Build history of the part. All positions in model axes, mm. A direction names the side the tool comes from. Coordinates: 2 decimals unless noted, no trailing zeros. Write each loop counter-clockwise with the first axis right and the second up, starting at its lowest first coordinate (ties: lowest second). Pieces come first, ordered by that corner, then holes.
```python
from build123d import *

# Parameters (mm, degrees)
SKETCH1_W                = 16.2
SKETCH1_H                = 8.4
BOSS_EXTRUDE1_DEPTH      = 14.5
SKETCH3_R                = 1.9
BOSS_EXTRUDE2_DEPTH      = 3
SKETCH3_3_R              = 1.9
BOSS_EXTRUDE3_DEPTH      = 6
SKETCH6_W                = 3.5
SKETCH6_H                = 8.4
SKETCH6_R                = 1
BOSS_EXTRUDE4_DEPTH      = 0.6
FILLET2_START            = -1
FILLET2_DEPTH            = 19
FILLET3_START            = -1
FILLET3_DEPTH            = 16
BOSS_EXTRUDE5_DEPTH      = 0.6
SKETCH8_W                = 3.8
SKETCH8_H                = 4
BOSS_EXTRUDE6_DEPTH      = 0.6
CHAMFER1_SIZE            = 1
M2_CLEARANCE_HOLE1_D     = 2.4
M2_CLEARANCE_HOLE1_DEPTH = 6
M2_CLEARANCE_HOLE1_TIP   = 0.721032743


with BuildPart() as part:
    # Sketch1 → Boss-Extrude1 (new body)
    with BuildSketch(Plane(origin=(0, 0, 0), x_dir=(1, 0, 0), z_dir=(0, 1, 0))):
        Rectangle(SKETCH1_W, SKETCH1_H)
    extrude(amount=BOSS_EXTRUDE1_DEPTH)

    # Sketch3 → Boss-Extrude2 (add)
    with BuildSketch(Plane(origin=(0, 14.5, 0), x_dir=(1, 0, 0), z_dir=(0, 1, 0))):
        with BuildLine():
            Line((3.9, 4.2), (8.1, 4.2))
            Line((8.1, 4.2), (8.1, -4.2))
            Line((8.1, -4.2), (3.9, -4.2))
            ThreePointArc((3.9, -4.2), (1.840026431, -3.660124164), (0.309638554, -2.179289951))
            ThreePointArc((0.309638554, -2.179289951), (-2.5, 0), (0.309638554, 2.179289951))
            ThreePointArc((0.309638554, 2.179289951), (1.840026431, 3.660124164), (3.9, 4.2))
        make_face()
        with Locations(Location((3.9, 0, 0), (0, 0, 270))):
            Circle(SKETCH3_R, mode=Mode.SUBTRACT)
    extrude(amount=BOSS_EXTRUDE2_DEPTH)

    # Sketch3<3> → Boss-Extrude3 (add)
    with BuildSketch(Plane(origin=(0, 14.5, 0), x_dir=(1, 0, 0), z_dir=(0, 1, 0))):
        with Locations(Location((3.9, 0, 0), (0, 0, 270))):
            Circle(SKETCH3_3_R)
    extrude(amount=BOSS_EXTRUDE3_DEPTH)

    # Sketch6 → Boss-Extrude4 (add)
    # profile 1 of 2: a face of its own
    with BuildSketch(Plane(origin=(0, 8, 0), x_dir=(1, 0, 0), z_dir=(0, 1, 0))):
        with Locations((9.85, 0)):
            Rectangle(SKETCH6_W, SKETCH6_H)
        with Locations(Location((9.75, 0, 0), (0, 0, 270))):
            Circle(SKETCH6_R, mode=Mode.SUBTRACT)
    # profile 2 of 2: a face of its own
    with BuildSketch(Plane(origin=(0, 8, 0), x_dir=(1, 0, 0), z_dir=(0, 1, 0))):
        with Locations((-9.85, 0)):
            Rectangle(SKETCH6_W, SKETCH6_H)
        with Locations(Location((-9.75, 0, 0), (0, 0, 90))):
            Circle(SKETCH6_R, mode=Mode.SUBTRACT)
    extrude(amount=BOSS_EXTRUDE4_DEPTH)

    # Fillet2: read off the stored shape, not the designer's step
    # Fillet2 outline → Fillet2 (cut)
    with BuildSketch(Plane(origin=(0, 0, 0), x_dir=(1, 0, 0), z_dir=(0, 1, 0)).offset(FILLET2_START)):
        with BuildLine():
            ThreePointArc((7.4, 4.2), (10.369848481, 2.969848481), (11.6, 0))
            Line((11.6, 0), (11.6, 4.2))
            Line((11.6, 4.2), (7.4, 4.2))
        make_face()
        with BuildLine():
            Line((11.6, -4.2), (11.6, 0))
            ThreePointArc((11.6, 0), (10.369848481, -2.969848481), (7.4, -4.2))
            Line((7.4, -4.2), (11.6, -4.2))
        make_face()
    extrude(amount=FILLET2_DEPTH, mode=Mode.SUBTRACT)

    # Fillet3: read off the stored shape, not the designer's step
    # Fillet3 outline → Fillet3 (cut)
    with BuildSketch(Plane(origin=(0, 0, 0), x_dir=(1, 0, 0), z_dir=(0, 1, 0)).offset(FILLET3_START)):
        with BuildLine():
            ThreePointArc((-7.4, -4.2), (-10.369848481, -2.969848481), (-11.6, 0))
            Line((-11.6, 0), (-11.6, -4.2))
            Line((-11.6, -4.2), (-7.4, -4.2))
        make_face()
        with BuildLine():
            Line((-11.6, 4.2), (-11.6, 0))
            ThreePointArc((-11.6, 0), (-10.369848481, 2.969848481), (-7.4, 4.2))
            Line((-7.4, 4.2), (-11.6, 4.2))
        make_face()
    extrude(amount=FILLET3_DEPTH, mode=Mode.SUBTRACT)

    # Sketch7 → Boss-Extrude5 (add)
    with BuildSketch(Plane(origin=(0, 17.5, 0), x_dir=(1, 0, 0), z_dir=(0, 1, 0))):
        with BuildLine():
            Line((-1.05, 1), (0.4, 1))
            ThreePointArc((0.4, 1), (1.4, 0), (0.4, -1))
            Line((0.4, -1), (-1.05, -1))
            ThreePointArc((-1.05, -1), (-2.05, 0), (-1.05, 1))
        make_face()
    extrude(amount=BOSS_EXTRUDE5_DEPTH)

    # Sketch8 → Boss-Extrude6 (add)
    with BuildSketch(Plane(origin=(8.1, 0, 0), x_dir=(0, 0, -1), z_dir=(1, 0, 0))):
        with Locations((0, 2)):
            Rectangle(SKETCH8_W, SKETCH8_H)
    extrude(amount=BOSS_EXTRUDE6_DEPTH)

    # Chamfer1
    chamfer1_edges = [part.edges().sort_by_distance(p)[0] for p in [
        (-8.1, 14.5, 0),
    ]]
    chamfer(chamfer1_edges, length=CHAMFER1_SIZE)

    # M2 Clearance Hole1
    with Locations(Plane(origin=(0, 20.5, 0), x_dir=(1, 0, 0), z_dir=(0, 1, 0))):
        with Locations((3.9, 0)):
            Hole(M2_CLEARANCE_HOLE1_D / 2, depth=M2_CLEARANCE_HOLE1_DEPTH)
            with Locations((0, 0, -(M2_CLEARANCE_HOLE1_DEPTH + M2_CLEARANCE_HOLE1_TIP / 2))):  # 118° drill point
                Cone(0, M2_CLEARANCE_HOLE1_D / 2, M2_CLEARANCE_HOLE1_TIP, mode=Mode.SUBTRACT)


solid = part.part
```
1. 3-axis set-ups, long thin cutter, end or side, ignore diameter. For faces 4 (the face through (8.7, 2, 0)), 5 (the face through (-8.1, 4, 0)), 6 (the face through (2.755, 17.458, -0.36)): which of +Z, -Z, +X, -X, +Y, -Y reach the whole face in a straight line?
Computed values:
face 4: +Z, -Z, +X, -Y
face 5: +Z, -Z, -X, -Y
face 6: +Y
2. Saw through at A-A on y = 2.25. List the corners of the cut face in (x, z).
Computed values:
outline: (-8.1, -4.14) arc R4.2 ccw to (-7.4, -4.2) - (7.4, -4.2) arc R4.2 ccw to (8.1, -4.14) - (8.1, -1.9) - (8.7, -1.9) - (8.7, 1.9) - (8.1, 1.9) - (8.1, 4.14) arc R4.2 ccw to (7.4, 4.2) - (-7.4, 4.2) arc R4.2 ccw to (-8.1, 4.14) - close
3. Mould opens along X. For faces 1 (the face through (8.1, 13, 0)), 2 (the face through (-2.05, 17.8, 0.02)), 3 (the face through (10.74, 8.3, -0.13)) say: +X half, -X half, draft (parallel to the pull), parting line (faces both ways), or undercut.
Computed values:
face 1: +X half
face 2: -X half
face 3: undercut
4. Saw through at D-D on z = -1.5. List the corners of the cut face in (x, y), plus the area to 3 significant figures.
Computed values:
outline: (-11.32, 8) - (-8.1, 8) - (-8.1, 0) - (8.7, 0) - (8.7, 4) - (8.1, 4) - (8.1, 8) - (11.32, 8) - (11.32, 8.6) - (8.1, 8.6) - (8.1, 17.5) - (5.07, 17.5) - (5.07, 20.5) - (2.73, 20.5) - (2.73, 17.5) - (-1.93, 17.5) - (-1.93, 14.5) - (-7.1, 14.5) - (-8.1, 13.5) - (-8.1, 8.6) - (-11.32, 8.6) - close
area: 278 mm2
5. Flat gauge pins, fed straight in: pin 1 (2 mm diameter, centred on x = -5, z = -3, fed in from -Y); pin 2 (1 mm diameter, centred on y = 12.5, z = 0, fed in from -X); pin 3 (1 mm diameter, centred on x = -10, z = 1, fed in from -Y); pin 4 (2.5 mm diameter, centred on x = -9.75, z = 0, fed in from +Y). Where does each tip first touch, or does it go through?
Computed values:
pin 1: stops at y = 0
pin 2: stops at x = -8.1
pin 3: stops at y = 8
pin 4: stops at y = 8.6
6. Probe line 1 along X through (y, z) = (10, 2.75); line 2 along Y through (x, z) = (2.25, -2); line 3 along Y through (x, z) = (-6, -0.5). List the from-to ranges inside material, lowest first.
Computed values:
line 1: x = -8.1 to 8.1
line 2: y = 0 to 17.5
line 3: y = 0 to 14.5
7. Saw through at B-B on x = -0.25. List the corners of the cut face in (y, z).
Computed values:
outline: (0, -4.2) - (14.5, -4.2) - (14.5, -2.25) - (17.5, -2.25) - (17.5, -1) - (18.1, -1) - (18.1, 1) - (17.5, 1) - (17.5, 2.25) - (14.5, 2.25) - (14.5, 4.2) - (0, 4.2) - close
8. Saw through at C-C on x = -9.75. List the corners of the cut face in (y, z), plus the area to 3 significant figures.
Computed values:
outline: (8, -3.48) - (8.6, -3.48) - (8.6, -1) - (8, -1) - close; (8, 1) - (8.6, 1) - (8.6, 3.48) - (8, 3.48) - close
area: 2.98 mm2
